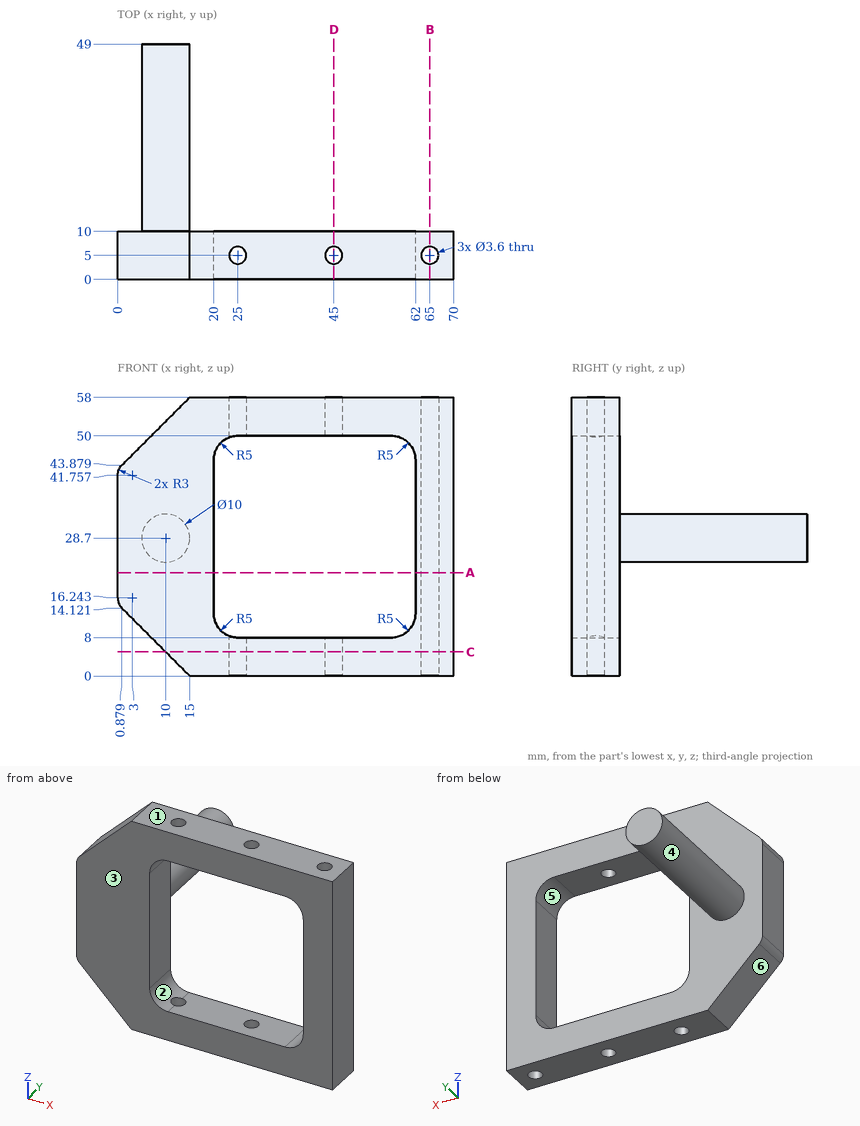
The figure shows three views and two pictorial views of one solid part (mm, origin at its lowest corner). Answer the questions. A direction names the side the tool comes from. Round coordinates to 2 decimals unless told otherwise and drop trailing zeros. Loops run counter-clockwise (first coordinate to the right, second up) from the corner with the lowest first, then second, coordinate; pieces in that order, holes last. Notation, with made-up numbers: M -38,22 L 2,22 A21 ccw 2,37 Z; hole C -14,-12.75 d2. An arc over 180 degrees is marked long. Use CSV: the item, a comma, the result in double quotes.
Q1. The mould has two halves that part along Z. Classify the marked faces 1, 2 and 3: pulls with the +Z half, pulls with the -Z half, needs draft (parallel to the pull), parting line crosses it, or undercut.
Determined:
face 1,"pulls with the +Z half"
face 2,"undercut"
face 3,"needs draft"
Q2. A tool of negligible diameter and unlimited length cuts with its end or side. For the marked faces 4, 5 and 6, from which of +Z, -Z, +X, -X, +Y, -Y can it reach the whole face along a straight path? Write none if from no direction.
Determined:
face 4,"+Y"
face 5,"+Y, -Y"
face 6,"-Z, -X, +Y, -Y"
Q3. Section A-A, the plane z = 21.5 is taken. Determine the outline of the cut face in (x, y).
Determined:
outline,"M 0,0 L 20,0 L 20,10 L 0,10 Z; M 62,0 L 70,0 L 70,10 L 62,10 Z; hole C 65,5 d3.6"
Q4. Each of these flat-tipped pins is pushed along its axis until it touches: pin 1 (5 mm diameter, centred on x = 9, z = 45.5, fed in from +Y); pin 2 (5 mm diameter, centred on x = 13.5, y = 31.5, fed in from -Z); pin 3 (8 mm diameter, centred on y = 38.5, z = 35, fed in from +X). Where does it stop, or does it pass through?
Determined:
pin 1,"y = 10"
pin 2,"z = 23.8"
pin 3,"x = 14.44"
Q5. Section D-D, the plane x = 45 is taken. Determine the outline of the cut face in (y, z), then the cut area to 3 significant figures.
Determined:
outline,"M 0,0 L 3.2,0 L 3.2,8 L 0,8 Z; M 0,50 L 3.2,50 L 3.2,58 L 0,58 Z; M 6.8,0 L 10,0 L 10,8 L 6.8,8 Z; M 6.8,50 L 10,50 L 10,58 L 6.8,58 Z"
area,"102 mm2"
Q6. Section B-B, the plane x = 65 is taken. Determine the outline of the cut face in (y, z), then the cut area to 3 significant figures.
Determined:
outline,"M 0,0 L 3.2,0 L 3.2,58 L 0,58 Z; M 6.8,0 L 10,0 L 10,58 L 6.8,58 Z"
area,"371 mm2"
Q7. Consider L1, parallel to X at y = 8, z = 29; L2, parallel to Z at x = 57, y = 7.5; L3, parallel to Y at x = 65, z = 18. Determine where each line is inside the solid, lowest interval first.
Determined:
L1,"0 to 20, 62 to 70"
L2,"0 to 8, 50 to 58"
L3,"0 to 3.2, 6.8 to 10"
Q8. Section C-C, the plane z = 5 is taken. Determine the outline of the cut face in (x, y).
Determined:
outline,"M 10,0 L 70,0 L 70,10 L 10,10 Z; hole C 25,5 d3.6; hole C 45,5 d3.6; hole C 65,5 d3.6"
